```python
from build123d import *

# Parameters (mm, degrees)
SKETCH1_W                      = 32
SKETCH1_H                      = 72
BOSS_EXTRUDE1_DEPTH            = 1.6
SKETCH2_R                      = 2.1
CUT_EXTRUDE1_DEPTH             = 79.807106279
LPATTERN1_COUNT                = 3
LPATTERN1_PITCH                = 8
LPATTERN1_COUNT_DIR2           = 9
LPATTERN1_PITCH_DIR2           = 8
EDGE_FLANGE1_STRIP_W           = 8.4
EDGE_FLANGE1_STRIP_H           = 1.6
EDGE_FLANGE1_STRIP_CUT_DEPTH   = 72
EDGE_FLANGE1_STRIP_2_W         = 8.4
EDGE_FLANGE1_STRIP_2_H         = 1.6
EDGE_FLANGE1_STRIP_CUT_2_DEPTH = 72
EDGE_FLANGE1_DEPTH             = 72
EDGE_FLANGE1_BEND_DEPTH        = 72
FILLET1_R                      = 5
SKETCH14_R                     = 2.1
CUT_EXTRUDE2_DEPTH             = 81.113981302
LPATTERN2_COUNT                = 9
LPATTERN2_PITCH                = 8


# Sheet-metal steps are written as plain solids
with BuildPart() as part:
    # Sketch1 → Boss-Extrude1 (new body)
    with BuildSketch(Plane(origin=(0, 0, 0), x_dir=(1, 0, 0), z_dir=(0, 1, 0))):
        with Locations((16, -36)):
            Rectangle(SKETCH1_W, SKETCH1_H)
    extrude(amount=BOSS_EXTRUDE1_DEPTH)

    # Sketch2 → Cut-Extrude1 (cut, through all)
    with BuildSketch(Plane(origin=(0, 1.6, 0), x_dir=(1, 0, 0), z_dir=(0, 1, 0))):
        with Locations(Location((8, -4, 0), (0, 0, 270))):
            Circle(SKETCH2_R)
    cut_extrude1 = extrude(amount=-CUT_EXTRUDE1_DEPTH, mode=Mode.SUBTRACT)

    # LPattern1: Cut-Extrude1 3 × 9
    with Locations(*[(i * LPATTERN1_PITCH, 0, j * LPATTERN1_PITCH_DIR2) for i in range(LPATTERN1_COUNT) for j in range(LPATTERN1_COUNT_DIR2) if (i, j) != (0, 0)]):
        add(cut_extrude1, mode=Mode.SUBTRACT)

    # Edge-Flange1 strip (across the edge) → Edge-Flange1 strip cut (cut)
    with BuildSketch(Plane(origin=(32, 1.6, 72), x_dir=(-1, 0, 0), z_dir=(0, 0, -1))):
        with Locations((-1.6, -0.8)):
            Rectangle(EDGE_FLANGE1_STRIP_W, EDGE_FLANGE1_STRIP_H)
    extrude(amount=EDGE_FLANGE1_STRIP_CUT_DEPTH, mode=Mode.SUBTRACT)

    # Edge-Flange1 strip 2 (across the edge) → Edge-Flange1 strip cut 2 (cut)
    with BuildSketch(Plane(origin=(0, 1.6, 0), x_dir=(1, 0, 0), z_dir=(0, 0, 1))):
        with Locations((-1.6, -0.8)):
            Rectangle(EDGE_FLANGE1_STRIP_2_W, EDGE_FLANGE1_STRIP_2_H)
    extrude(amount=EDGE_FLANGE1_STRIP_CUT_2_DEPTH, mode=Mode.SUBTRACT)

    # Edge-Flange1 section (across the edge) → Edge-Flange1 (add)
    with BuildSketch(Plane(origin=(32, 1.6, 72), x_dir=(-1, 0, 0), z_dir=(0, 0, -1))):
        with BuildLine():
            Line((0, 1), (0, 12.9))
            Line((0, 12.9), (1.6, 12.9))
            Line((1.6, 12.9), (1.6, 1))
            ThreePointArc((1.6, 1), (1.892893219, 0.292893219), (2.6, 0))
            Line((2.6, 0), (2.6, -1.6))
            ThreePointArc((2.6, -1.6), (0.761522369, -0.838477631), (0, 1))
        make_face()
    extrude(amount=EDGE_FLANGE1_DEPTH)

    # Edge-Flange1 section 2 (across the edge) → Edge-Flange1 bend (add)
    with BuildSketch(Plane(origin=(0, 1.6, 0), x_dir=(1, 0, 0), z_dir=(0, 0, 1))):
        with BuildLine():
            Line((0, 1), (0, 12.9))
            Line((0, 12.9), (1.6, 12.9))
            Line((1.6, 12.9), (1.6, 1))
            ThreePointArc((1.6, 1), (1.892893219, 0.292893219), (2.6, 0))
            Line((2.6, 0), (2.6, -1.6))
            ThreePointArc((2.6, -1.6), (0.761522369, -0.838477631), (0, 1))
        make_face()
    extrude(amount=EDGE_FLANGE1_BEND_DEPTH)

    # Fillet1
    fillet1_edges = [part.edges().sort_by_distance(p)[0] for p in [
        (31.2, 14.5, 72),
        (31.2, 14.5, 0),
        (0.8, 14.5, 0),
        (0.8, 14.5, 72),
    ]]
    fillet(fillet1_edges, radius=FILLET1_R)

    # Sketch14 → Cut-Extrude2 (cut, through all)
    with BuildSketch(Plane.ZY):
        with Locations(Location((4, 8.1, 0), (0, 0, 270))):
            Circle(SKETCH14_R)
    cut_extrude2 = extrude(amount=-CUT_EXTRUDE2_DEPTH, mode=Mode.SUBTRACT)

    # LPattern2: Cut-Extrude2 ×9
    with Locations(*[(0, 0, i * LPATTERN2_PITCH) for i in range(1, LPATTERN2_COUNT)]):
        add(cut_extrude2, mode=Mode.SUBTRACT)


solid = part.part
```
Geometry check sheet. Reference: the model listing, model coordinates, mm. A direction names the side the tool comes from. Coordinates: 2 decimals unless noted, no trailing zeros.
Item 1: Go/stop test with a flat-tipped pin: pin 1 Ø4 at (x, z) = (15.5, 29.5) entering from +Y. Record where the tip stops, or that it passes through.
Item 2: Sectioned sample at A-A, the plane z = 45. Count the separate pieces of the cut face and the enclosed holes in it, then the cut area to 3 significant figures.
Item 3: Release check for a two-part mould opening along Z. For faces 3 (the face through (31.19, 8.56, 41.95)), 4 (the face through (1, 14.5, 36)), 5 (the face through (0.81, 13.07, 1.5)) record: released by +Z, released by -Z, zero draft, split by the parting line, or undercut.
Item 4: Access from +Z, -Z, +X, -X, +Y, -Y to the whole of each face (thin tool, end or side, straight path). Record for faces 1 (the face through (30.4, 11, 37)), 2 (the face through (10.082, 0.811, 43.727)).
Item 5: Thickness scan on line 1 (X direction, y = 13.5, z = 51); line 2 (X direction, y = 1, z = 20); line 3 (Y direction, x = 13, z = 67.5). Record the ranges inside material, lowest first.
Check result:
1. pin 1: stops at y = 1.6
2. separate pieces: 6
2. enclosed holes: 0
2. area: 60.5 mm2
3. face 3: undercut
3. face 4: zero draft
3. face 5: released by -Z
4. face 1: +Z, -Z, +Y
4. face 2: +Y, -Y
5. line 1: x = 0 to 1.6, 30.4 to 32
5. line 2: x = 0.55 to 5.9, 10.1 to 13.9, 18.1 to 21.9, 26.1 to 31.45
5. line 3: y = 0 to 1.6
